Work out the finished part from the listing and answer in its coordinate system (mm). A direction names the side the tool comes from. Give positions to 0.01 mm unless a question says otherwise; leave off trailing zeros. Order: outer loops, then holes, each group sorted by start corner. A loop starts at its lowest first (then second) coordinate and runs counter-clockwise, first axis right, second up. Notation, with made-up numbers: (21, 67.25) - (52, 67.25) arc R19 cw to (52, 96.25) - close; hole circle Ø6 at (-0.5, -11.75). An arc over 180 degrees is marked (long way). Write each question's results on one line, items separated by ' | '.
Autodesk Inventor part; units mm, degrees
ref_plane "YZ Plane" through (0, 0, 0) normal (1, 0, 0) x (0, 1, 0)
ref_plane "XZ Plane" through (0, 0, 0) normal (0, 1, 0) x (-1, 0, 0)
ref_plane "XY Plane" through (0, 0, 0) normal (0, 0, 1) x (1, 0, 0)
sketch "Boceto1" plane through (0, 0, 0) normal (0, 1, 0) x (-1, 0, 0)
  line L0 (-122.5, 35) -> (122.5, 35)
  line L1 (122.5, 35) -> (122.5, -35)
  line L2 (122.5, -35) -> (-122.5, -35)
  line L3 (-122.5, -35) -> (-122.5, 35)
  line L4 (-122.5, 35) -> (122.5, -35) construction
  line L5 (122.5, 35) -> (-122.5, -35) construction
  point P0 (0, 0)
  dimension "d0" = 245
  dimension "d1" = 70
extrude "Extrusión1" add sketch "Boceto1" along normal blind 25.4
sketch "Boceto2" plane through (0, 0, 0) normal (0, -1, 0) x (1, 0, 0)
  line L0 (-109.8, 33.98) -> (109.8, 33.98)
  line L1 (109.8, -33.98) -> (-109.8, -33.98)
  line L2 (-109.8, -33.98) -> (-109.8, 33.98)
  line L3 (109.8, 33.98) -> (109.8, -33.98)
  line L4 (-122.5, -35) -> (-122.5, 35)
  line L5 (-122.5, 35) -> (122.5, 35)
  dimension "d8" = 12.7
  dimension "d9" = 1.02
extrude "Extrusión2" cut sketch "Boceto2" against normal blind 24.38
sketch "Boceto3" plane through (-109.8, 0, 33.98) normal (1, 0, 0) x (0, 0, -1)
  line L0 (-1.02, 0) -> (-1.02, 25.4) construction
  line L1 (68.98, 0) -> (68.98, 25.4) construction
  circle A0 centre (6.5, 6.35) radius 4.7625
  line L2 (0, 0) -> (0, 24.38)
  line L3 (67.96, 0) -> (0, 0)
  circle A1 centre (17.5, 6.35) radius 4.7625
  circle A2 centre (28.5, 6.35) radius 4.7625
  circle A3 centre (39.5, 6.35) radius 4.7625
  circle A4 centre (50.5, 6.35) radius 4.7625
  circle A5 centre (61.5, 6.35) radius 4.7625
  point P0 (33.98, 0)
  dimension "d12" = 9.525
  dimension "d13" = 6.5
  dimension "d14" = 6.35
  dimension "d17" = 11
extrude "Extrusión3" add sketch "Boceto3" along normal up to surface (219.6 mm away)
sketch "Boceto4" plane through (0, 25.4, 0) normal (0, 1, 0) x (1, 0, 0)
  line L0 (-122.5, 35) -> (-73.5, 35) construction
  line L1 (-73.5, 35) -> (-73.5, -35) construction
  line L2 (-122.5, -35) -> (122.5, -35) construction
  line L3 (-122.5, -35) -> (-73.5, 35) construction
  line L4 (-122.5, 35) -> (-73.5, -35) construction
  line L5 (122.5, 35) -> (-122.5, 35) construction
  line L6 (122.5, 35) -> (73.5, 35) construction
  line L7 (73.5, 35) -> (73.5, -35) construction
  line L8 (73.5, -35) -> (122.5, 35) construction
  line L9 (73.5, 35) -> (122.5, -35) construction
  circle A0 centre (-98, 0) radius 3.175
  circle A1 centre (98, 0) radius 3.175
  point P0 (0, 0)
  dimension "d24" = 49
  dimension "d25" = 49
  dimension "d26" = 6.35
  dimension "d27" = 6.35
extrude "Extrusión4" add sketch "Boceto4" along normal blind 19.05
thread "Rosca1"
thread "Rosca2"
chamfer "Chaflán1" distance 0.5 angle 45 1 edges at (-101.175, 44.45, 0)
chamfer "Chaflán2" distance 0.5 angle 45 1 edges at (94.825, 44.45, 0)
sketch "Boceto5" plane through (0, 25.4, 0) normal (0, 1, 0) x (1, 0, 0)
  line L0 (-122.5, -35) -> (122.5, -35) construction
  line L1 (-109.8, -35) -> (-109.8, 35.0447) construction
  line L2 (-122.5, 35) -> (-122.5, -35) construction
  line L3 (-109.8, -35) -> (-109.8, -17.489) construction
  line L4 (-109.8, -11.7175) -> (-109.8, -21.2425) construction
  line L5 (-109.8, 35.0447) -> (-109.8, 17.5337) construction
  line L6 (-109.8, 33.98) -> (-109.8, -33.98) construction
  circle A0 centre (-109.8, -17.489) radius 3.175
  circle A1 centre (-109.8, 17.5337) radius 3.175
  circle A2 centre (-109.8, -17.489) radius 3.685
  circle A3 centre (-109.8, 17.5337) radius 3.685
  point P0 (0, 0)
  dimension "d40" = 12.7
  dimension "d41" = 17.511
  dimension "d42" = 17.511
  dimension "d43" = 6.35
  dimension "d44" = 6.35
  dimension "d45" = 7.37
  dimension "d46" = 7.37
extrude "Extrusión5" add sketch "Boceto5" along normal blind 2
chamfer "Chaflán3" distance 0.5 angle 45 2 edges at (-113.485, 27.4, -17.5337) (-113.485, 27.4, 17.489)
sketch "Boceto6" plane through (-109.8, 25.4, 17.489) normal (0, 1, 0) x (1, 0, 0)
  circle A0 centre (0, 0) radius 3.175
sketch "Boceto7" plane through (-109.8, 25.4, -17.5337) normal (0, 1, 0) x (1, 0, 0)
  circle A0 centre (0, 0) radius 3.175
properties part number "resistencia_cuarzo_250-300W"
1. A tool of negligible diameter and unlimited length cuts with its end or side. For faces 1 (the face through (-1.54, 3.13, 8.99)), 2 (the face through (-110, 25.4, 18)), 3 (the face through (-2, 12, 33.98)), from which of +Z, -Z, +X, -X, +Y, -Y can it reach the whole face along a straight path? Write none if from no direction.
Answer list:
face 1: none | face 2: +Y | face 3: -Y
2. Straight lines are drawn through the part: line 1 (Z direction, x = -109.8, y = 26.25); line 2 (Y direction, x = 49, z = -27.5); line 3 (X direction, y = 19, z = -2). For each, find the intervals that lie inside material, in ascending order. Write a range as [from, to].
Answer list:
line 1: [-21.22, -20.71], [-14.36, -13.85], [13.8, 14.31], [20.66, 21.17] | line 2: [1.59, 11.11], [24.38, 25.4] | line 3: [-122.5, -109.8], [109.8, 122.5]
3. A cutting plane is placed at A-A, the plane z = 5.48. Write down the section's boundary in (x, y).
Answer list:
outline: (-122.5, 0) - (-109.8, 0) - (-109.8, 1.59) - (109.8, 1.59) - (109.8, 0) - (122.5, 0) - (122.5, 25.4) - (-122.5, 25.4) - close; hole (-109.8, 11.11) - (109.8, 11.11) - (109.8, 24.38) - (-109.8, 24.38) - close
4. A cutting plane is placed at C-C, the plane y = 14. Write down the section's boundary in (x, z), then the cut area to 3 significant figures.
Answer list:
outline: (-122.5, -35) - (122.5, -35) - (122.5, 35) - (-122.5, 35) - close; hole (-109.8, -33.98) - (109.8, -33.98) - (109.8, 33.98) - (-109.8, 33.98) - close | area: 2,230 mm^2
5. Given P1, Ø1.9, axis at x = -109, z = 16.5, coming from the +Y side; P2, Ø12, axis at x = -74, z = 11.5, coming from the -Y side; P3, Ø7.5, axis at x = -109.8, z = 17.489, coming from the +Y side; P4, Ø1, axis at x = 93.5, y = 29, coming from the -Z side, each flat-ended and moving along its own axis, determine where each tip first touches the part or whether it passes through.
Answer list:
P1: y = 25.4 | P2: y = 1.59 | P3: y = 27.4 | P4: through
6. Determine the mould class of faces 4 (the face through (-110, 25.4, -17)), 5 (the face through (-2, 24.38, 0)), 6 (the face through (-106.77, 26.39, -16.58)) for opening direction Y: +Y half, -Y half, draft (parallel to the pull), parting line (faces both ways), or undercut.
Answer list:
face 4: +Y half | face 5: undercut | face 6: draft
7. A cutting plane is placed at B-B, the plane x = -11. State how many separate pieces and enclosed holes the cut face has, then the cut area to 3 significant figures.
Answer list:
separate pieces: 7 | enclosed holes: 0 | area: 549 mm^2
